Geometry: final body of the model. Coordinates: model frame, mm. A direction names the side the tool comes from. Coordinates: 2 decimals unless noted, no trailing zeros. Loops run counter-clockwise (first coordinate to the right, second up) from the corner with the lowest first, then second, coordinate; pieces in that order, holes last. Notation, with made-up numbers: (36.5, 29) -> (56.5, 29) arc R14 cw to (56.5, 55) -> close; hole circle Ø2 at (65, 16.25). An arc over 180 degrees is marked (long way). One line per item, written item: value. Start each with the question number.
Item 1: Mould query, pull axis Z, two halves, no side actions, for faces 1 (the cylindrical face through (-12.508, -10.306, 24.756)), 2 (the flat face through (0, 35.56, 34)), 3 (the conical face through (-9.48, -2, 30.12)). Classes: +Z half, -Z half, draft (parallel to the pull), parting line (faces both ways), or undercut.
Item 2: Set-up query: faces 4 (the flat face through (31, 37.06, 8)), 5 (the flat face through (2.5, 36.6, 34.9)), 6 (the flat face through (0, -14.25, 13)), 7 (the flat face through (17, 39.31, -31)), 8 (the flat face through (-25, -6.25, 0)). Return all of +Z, -Z, +X, -X, +Y, -Y with unobstructed straight access to the full face (end or side cutting, diameter ignored); none if empty.
Item 3: Ray query, probe 1 along Y at (x, z) = (-8, -11); probe 2 along Y at (x, z) = (-5, 22); probe 3 along X at (y, z) = (16, -8). Return the intervals inside material, ascending. Write a range as from..to.
Item 4: Contact query for flat-ended pins moving along their axis: pin 1 Ø8 at (y, z) = (33, 17.5) entering from +X; pin 2 Ø10 at (y, z) = (22.5, -11) entering from +X; pin 3 Ø6 at (x, y) = (5, 11) entering from +Z. Output: stop coordinate, or through.
Item 5: Section query A-A on y = 14. Return loops of the section in (x, z) (1 decimal), then the cut area to 3 significant figures.
from build123d import *

# Parameters (mm, degrees)
CHAMFER1_SIZE     = 1.5
WIRE_START        = -3.75
SKETCH8_W         = 5
SKETCH8_H         = 8.104217416
WIRE_HOLE_DEPTH   = 3.75
SKETCH9_R         = 0.875
FRONT_HOLES_DEPTH = 6
SKETCH10_R        = 2.875
BACK_HOLES_DEPTH  = 8


with BuildPart() as part:
    # Sketch7 → Base Motor Housing (revolve)
    with BuildSketch(Plane.XY, mode=Mode.PRIVATE) as base_motor_housing_sk:
        Polygon((-38.0375, 39.31), (-35.0375, 39.31), (-35.0375, 37.06), (-30.0375, 37.06), (-30.0375, 4.505), (-29.2875, 4.505), (-29.2875, 1.25), (-20.0375, 1.25), (-12.5, -1.25), (-12.5, -14.25), (-38.0375, -14.25), align=None)
    revolve(base_motor_housing_sk.sketch.rotate(Axis((0, -30.231871117, 0), (0, 1, 0)), 270), axis=Axis((0, -30.231871117, 0), (0, 1, 0)))

    # Chamfer1
    chamfer1_edges = [part.edges().sort_by_distance(p)[0] for p in [
        (0, 37.06, 30.0375),
    ]]
    chamfer(chamfer1_edges, length=CHAMFER1_SIZE)

    # Sketch8 → Wire Hole (cut)
    with BuildSketch(Plane(origin=(0, 39.31, 0), x_dir=(1, 0, 0), z_dir=(0, 1, 0)).offset(WIRE_START)):
        with Locations((0, -33.985391292)):
            Rectangle(SKETCH8_W, SKETCH8_H)
    extrude(amount=WIRE_HOLE_DEPTH, mode=Mode.SUBTRACT)

    # Sketch9 → Front-Holes (cut)
    with BuildSketch(Plane(origin=(0, 37.06, 0), x_dir=(1, 0, 0), z_dir=(0, 1, 0))):
        with Locations(Location((-33.2875, 0, 0), (0, 0, 270))):
            Circle(SKETCH9_R)
        with Locations(Location((-16.64375, 28.827820628, 0), (0, 0, 270))):
            Circle(SKETCH9_R)
        with Locations(Location((16.64375, 28.827820628, 0), (0, 0, 270))):
            Circle(SKETCH9_R)
        with Locations(Location((33.2875, 0, 0), (0, 0, 270))):
            Circle(SKETCH9_R)
        with Locations(Location((16.64375, -28.827820628, 0), (0, 0, 270))):
            Circle(SKETCH9_R)
        with Locations(Location((-16.64375, -28.827820628, 0), (0, 0, 270))):
            Circle(SKETCH9_R)
    extrude(amount=-FRONT_HOLES_DEPTH, mode=Mode.SUBTRACT)

    # Sketch10 → Back-Holes (cut)
    with BuildSketch(Plane.XZ.offset(14.25)):
        with Locations(Location((-25.26875, 0, 0), (0, 0, 270))):
            Circle(SKETCH10_R)
        with Locations(Location((-12.634375, 21.883379422, 0), (0, 0, 270))):
            Circle(SKETCH10_R)
        with Locations(Location((12.634375, 21.883379422, 0), (0, 0, 270))):
            Circle(SKETCH10_R)
        with Locations(Location((25.26875, 0, 0), (0, 0, 270))):
            Circle(SKETCH10_R)
        with Locations(Location((12.634375, -21.883379422, 0), (0, 0, 270))):
            Circle(SKETCH10_R)
        with Locations(Location((-12.634375, -21.883379422, 0), (0, 0, 270))):
            Circle(SKETCH10_R)
    extrude(amount=-BACK_HOLES_DEPTH, mode=Mode.SUBTRACT)

    # Sketch11 → Cut-Revolve1 (revolve, cut)
    with BuildSketch(Plane.XY, mode=Mode.PRIVATE) as cut_revolve1_sk:
        Polygon((31.14375, -14.25), (31.14375, -2.25), (38.0375, 1.730108418), (38.0375, -14.25), align=None)
    revolve(cut_revolve1_sk.sketch.rotate(Axis((0, 0, 0), (0, -1, 0)), 90), axis=Axis((0, 0, 0), (0, -1, 0)), mode=Mode.SUBTRACT)


solid = part.part
Reply:
1. face 1: undercut
1. face 2: draft
1. face 3: parting line
2. face 4: +Y
2. face 5: +Z, +Y
2. face 6: +Z, -Z, +X, -X, -Y
2. face 7: +Z, -Z, +X, -X, +Y
2. face 8: -Y
3. probe 1: y = -14.25..-0.88
3. probe 2: y = -14.25..1.25
3. probe 3: x = -37.19..-28.95, 28.95..37.19
4. pin 1: stops at x = 35.56
4. pin 2: stops at x = 37.56
4. pin 3: stops at z = 37.98
5. outline: circle Ø76.1 at (0, 0); hole circle Ø60.1 at (0, 0)
5. area: 1,710 mm²
